from build123d import *

# Parameters (mm, degrees)
BOSS_EXTRUDE1_DEPTH = 38.1
SKETCH2_R           = 3.556
CUT_EXTRUDE1_DEPTH  = 7.35
SKETCH3_R           = 3.556
CUT_EXTRUDE2_DEPTH  = 7.35
FILLET1_R           = 22.86
FILLET2_R           = 2.54
CHAMFER1_SIZE       = 6.35


with BuildPart() as part:
    # Sketch1 → Boss-Extrude1 (new body)
    with BuildSketch(Plane(origin=(0, 0, 0), x_dir=(1, 0, 0), z_dir=(0, 1, 0))):
        Polygon((0, 0), (0, -76.2), (6.35, -76.2), (6.35, -6.35), (76.2, -6.35), (76.2, 0), align=None)
    extrude(amount=BOSS_EXTRUDE1_DEPTH)

    # Sketch2 → Cut-Extrude1 (cut, through all)
    with BuildSketch(Plane(origin=(6.35, 0, 0), x_dir=(0, 0, -1), z_dir=(1, 0, 0))):
        with Locations((-38.1, 19.05)):
            Circle(SKETCH2_R)
    extrude(amount=-CUT_EXTRUDE1_DEPTH, mode=Mode.SUBTRACT)

    # Sketch3 → Cut-Extrude2 (cut, through all)
    with BuildSketch(Plane.XY.offset(6.35)):
        with Locations((38.1, 19.05)):
            Circle(SKETCH3_R)
    extrude(amount=-CUT_EXTRUDE2_DEPTH, mode=Mode.SUBTRACT)

    # Fillet1
    fillet1_edges = [part.edges().sort_by_distance(p)[0] for p in [
        (6.35, 19.05, 6.35),
    ]]
    fillet(fillet1_edges, radius=FILLET1_R)

    # Fillet2
    fillet2_edges = [part.edges().sort_by_distance(p)[0] for p in [
        (76.2, 19.05, 6.35),
        (6.35, 19.05, 76.2),
        (6.35, 38.1, 52.705),
        (52.705, 0, 6.35),
        (52.705, 38.1, 6.35),
        (13.045538982, 0, 13.045538982),
        (13.045538982, 38.1, 13.045538982),
        (6.35, 0, 52.705),
    ]]
    fillet(fillet2_edges, radius=FILLET2_R)

    # Chamfer1
    chamfer1_edges = [part.edges().sort_by_distance(p)[0] for p in [
        (0, 19.05, 0),
    ]]
    chamfer(chamfer1_edges, length=CHAMFER1_SIZE)


solid = part.part
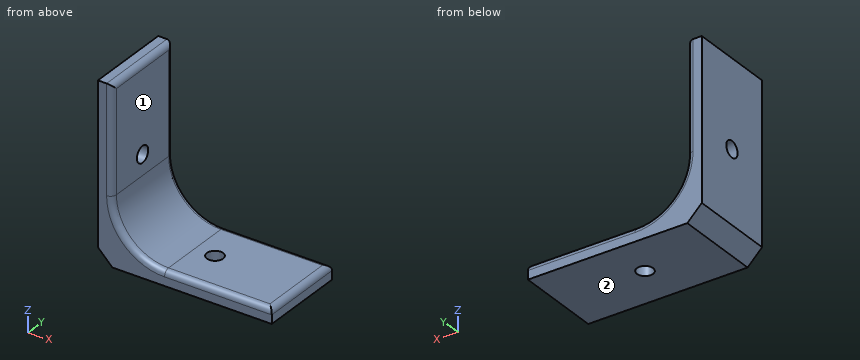
Input: part model. Units: mm. Frame: model coordinates. Face numbers are marked on the shaded views. A direction names the side the tool comes from. Round coordinates to 2 decimals unless told otherwise and drop trailing zeros. Write each loop counter-clockwise with the first axis right and the second up, starting at its lowest first coordinate (ties: lowest second). Pieces come first, ordered by that corner, then holes.
1) Contact query for flat-ended pins moving along their axis: P1, Ø16.5, axis at x = 47.5, y = 18.5, coming from the +Z side; P2, Ø11.5, axis at y = 19.05, z = 38.1, coming from the +X side; P3, Ø5, axis at x = 30.5, y = 30, coming from the +Z side. Output: stop coordinate, or through.
2) Cut plane A-A (y = 19.05). Return the cut outline in (x, z).
3) Ray query, L1, parallel to Y at x = 4, z = 38.1; L2, parallel to X at y = 3, z = 61; L3, parallel to X at y = 19, z = 4. Return the intervals inside material, ascending.
4) Cut plane B-B (x = 38.1). Return the cut outline in (y, z).
5) Cut plane C-C (z = 38.1). Return the cut outline in (x, y).
6) Reachability of the marked faces 1 and 2 from +Z, -Z, +X, -X, +Y, -Y: full face, straight path, thin tool, end or side. Return the list, or none.
7) Cut plane D-D (y = 28.5). Return the cut outline in (x, z).
Geometry says:
1. P1: stops at z = 6.35
1. P2: stops at x = 6.35
1. P3: stops at z = 6.38
2. outline: (0, 6.35) - (6.35, 0) - (34.54, 0) - (34.54, 6.35) - (29.21, 6.35) arc R22.86 cw to (6.35, 29.21) - (6.35, 34.54) - (0, 34.54) - close; (0, 41.66) - (6.35, 41.66) - (6.35, 73.66) arc R2.54 ccw to (3.81, 76.2) - (0, 76.2) - close; (41.66, 0) - (76.2, 0) - (76.2, 3.81) arc R2.54 ccw to (73.66, 6.35) - (41.66, 6.35) - close
3. L1: y = 0.01 to 15.49, 22.61 to 38.09
3. L2: x = 0 to 6.35
3. L3: x = 2.35 to 34.54, 41.66 to 76.19
4. outline: (0, 0) - (15.49, 0) - (15.49, 6.35) - (2.54, 6.35) arc R2.54 ccw to (0, 3.81) - close; (22.61, 0) - (38.1, 0) - (38.1, 3.81) arc R2.54 ccw to (35.56, 6.35) - (22.61, 6.35) - close
5. outline: (0, 0) - (3.81, 0) arc R2.54 ccw to (6.35, 2.54) - (6.35, 15.49) - (0, 15.49) - close; (0, 22.61) - (6.35, 22.61) - (6.35, 35.56) arc R2.54 ccw to (3.81, 38.1) - (0, 38.1) - close
6. face 1: +Z, +X, +Y, -Y
6. face 2: -Z, +X, -X, +Y, -Y
7. outline: (0, 6.35) - (6.35, 0) - (76.2, 0) - (76.2, 3.81) arc R2.54 ccw to (73.66, 6.35) - (29.21, 6.35) arc R22.86 cw to (6.35, 29.21) - (6.35, 73.66) arc R2.54 ccw to (3.81, 76.2) - (0, 76.2) - close
